from build123d import *

# Parameters (mm, degrees)
SCHNITT_LINEAR_AUSTRAGEN1_DEPTH = 4


with BuildPart() as part:
    # Skizze1 → Rotation1 (revolve)
    with BuildSketch(Plane(origin=(0, 0, 0), x_dir=(0, 0, -1), z_dir=(1, 0, 0))):
        Polygon((-4, 0), (-4, 4), (250.3, 4), (250.3, 10), (255.3, 10), (255.3, 0), align=None)
    revolve(axis=Axis((0, 0, -255.3), (0, 0, 1)))

    # Skizze2 → Rotation2 (revolve)
    with BuildSketch(Plane(origin=(0, 0, 0), x_dir=(0, 0, -1), z_dir=(1, 0, 0))):
        with BuildLine():
            Line((-24, 0), (-24, 3.233))
            Line((-24, 3.233), (-23.233, 4))
            Line((-23.233, 4), (-7.697981936, 4))
            Line((-7.697981936, 4), (-5.599415898, 3.236184428))
            ThreePointArc((-5.599415898, 3.236184428), (-5.498392718, 3.209115348), (-5.394203812, 3.2))
            Line((-5.394203812, 3.2), (-4.6, 3.2))
            ThreePointArc((-4.6, 3.2), (-4.175735931, 3.375735931), (-4, 3.8))
            Line((-4, 3.8), (-4, 4))
            Line((-4, 4), (-3, 4))
            Line((-3, 4), (-3, 0))
            Line((-3, 0), (-24, 0))
        make_face()
    revolve(axis=Axis((0, 0, 3), (0, 0, 1)))

    # Skizze3 → Schnitt-Linear austragen1 (cut)
    with BuildSketch(Plane.XY.offset(1)):
        Polygon((-7, 14), (-7, -7), (-3.5, -7), (-3.5, 7), (3.5, 7), (3.5, -7), (7, -7), (7, 14), align=None)
    extrude(amount=SCHNITT_LINEAR_AUSTRAGEN1_DEPTH, mode=Mode.SUBTRACT)


solid = part.part
Part model, mm, in its own coordinate system. Give positions to 0.01 mm unless a question says otherwise; leave off trailing zeros. Loops run counter-clockwise (first coordinate to the right, second up) from the corner with the lowest first, then second, coordinate; pieces in that order, holes last.
(1) Band-saw the part on B-B (z = -114.5). Write the cut outline in (x, y).
Return value:
outline: circle Ø8 at (0, 0)
(2) Pin check, flat tips, straight feed: pin 1 (10 mm diameter, centred on y = 0, z = -121, fed in from +X); pin 2 (8 mm diameter, centred on y = 6, z = -79, fed in from +X); pin 3 (2 mm diameter, centred on y = -4.5, z = -18, fed in from +X). Stop position of each tip, or through.
Return value:
pin 1: stops at x = 4
pin 2: stops at x = 3.46
pin 3: stops at x = 1.94
(3) Band-saw the part on C-C (y = 6.5). Write the cut outline in (x, z).
Return value:
outline: (-7.6, -255.3) - (7.6, -255.3) - (7.6, -250.3) - (-7.6, -250.3) - close
(4) Drill centre lines: line 1 along Z through (x, y) = (6, 3.5); line 2 along Y through (x, z) = (3.5, -61); line 3 along X through (y, z) = (-0.5, -126). Where is each one in solid material? Low to high.
Return value:
line 1: z = -255.3 to -250.3
line 2: y = -1.94 to 1.94
line 3: x = -3.97 to 3.97
(5) Band-saw the part on A-A (x = 0). Write the cut outline in (y, z).
Return value:
outline: (-10, -255.3) - (10, -255.3) - (10, -250.3) - (4, -250.3) - (4, 4) - (3.8, 4) arc R0.6 cw to (3.2, 4.6) - (3.2, 5.39) arc R0.6 cw to (3.24, 5.6) - (4, 7.7) - (4, 23.23) - (3.23, 24) - (-3.23, 24) - (-4, 23.23) - (-4, 7.7) - (-3.24, 5.6) arc R0.6 cw to (-3.2, 5.39) - (-3.2, 4.6) arc R0.6 cw to (-3.8, 4) - (-4, 4) - (-4, -250.3) - (-10, -250.3) - close
(6) Pull direction Z, two halves, no side cores. Call faces 1 (the cylindrical face through (1.947, -2.539, 4.992)), 2 (the flat face through (0, 0, -255.3)), 3 (the cylindrical face through (9.76, -2.17, -252.84)), 4 (the flat face through (0, 0, 24)): pulls with the +Z half, pulls with the -Z half, needs draft (parallel to the pull), parting line crosses it, or undercut.
Return value:
face 1: undercut
face 2: pulls with the -Z half
face 3: needs draft
face 4: pulls with the +Z half
